The listing builds one solid part. Answer for the finished solid, in the listing's coordinates (mm). Face numbers are marked on the shaded views. A direction names the side the tool comes from. Give positions to 0.01 mm unless a question says otherwise; leave off trailing zeros. Loops run counter-clockwise (first coordinate to the right, second up) from the corner with the lowest first, then second, coordinate; pieces in that order, holes last.
Item 1: Section A-A, the plane x = 3 is taken. Give the vertices of the cut face in (y, z).
Item 2: Each of these flat-tipped pins is pushed along its axis until it touches: pin 1 Ø1 at (y, z) = (-10.5, -11.5) entering from -X; pin 2 Ø2 at (x, y) = (-3, 6.5) entering from +Z; pin 3 Ø3 at (x, z) = (-3.5, -9.5) entering from -Y; pin 4 Ø5 at (x, y) = (0, -9) entering from -Z. Where does it stop, or does it pass through?
Item 3: A tool of negligible diameter and unlimited length cuts with its end or side. For the marked faces 1 and 2, from which of +Z, -Z, +X, -X, +Y, -Y can it reach the whole face along a straight path? Write none if from no direction.
Item 4: The mould has two halves that part along Y. Classify the marked faces 3 and 4: pulls with the +Y half, pulls with the -Y half, needs draft (parallel to the pull), parting line crosses it, or undercut.
Item 5: Consider line 1 along Z through (x, y) = (1, 0); line 2 along X through (y, z) = (-9, 8.5); line 3 along Y through (x, z) = (2, 3). Determine where each line is inside the solid, lowest interval first.
Item 6: Section B-B, the plane z = 4 is taken. Give the number of separate pieces and of enclosed holes in the cut face, and give its area (3 significant figures).
Autodesk Inventor part; units mm, degrees
ref_plane "body_screw_XY" through (0, -9, 5) normal (0, 0, 1) x (1, 0, 0)
ref_plane "body_screw_YZ" through (0, -9, 5) normal (1, 0, 0) x (0, 1, 0)
ref_plane "body_screw_ZX" through (0, -9, 5) normal (0, 1, 0) x (0, 0, 1)
sketch "Sketch_1" plane through (0, 0, 0) normal (0, 0, 1) x (1, 0, 0)
  line L0 (5, 0) -> (-5, 0)
  line L1 (-5, 14.5) -> (-5, 5.5)
  line L2 (-5, 5.5) -> (-4.5, 5)
  line L3 (-4.5, 5) -> (4.5, 5)
  line L4 (4.5, 5) -> (5, 5.5)
  line L5 (5, 5.5) -> (5, 14.5)
  line L6 (5, 14.5) -> (4.5, 15)
  line L7 (4.5, 15) -> (-4.5, 15)
  line L8 (-4.5, 15) -> (-5, 14.5)
revolve "Revolution1" add sketch "Sketch_1" angle 360 about axis through (5, 0, 0) along (1, 0, 0)
sketch "Sketch_2" plane through (0, 0, 0) normal (1, 0, 0) x (0, 1, 0)
  line L0 (-15, 0.75) -> (-15, -0.75)
  line L1 (-15, -0.75) -> (9, -0.75)
  line L2 (9, -0.75) -> (9, 0.75)
  line L3 (9, 0.75) -> (-15, 0.75)
extrude "Extrusion1" cut sketch "Sketch_2" along normal mid plane 10
sketch "Sketch_3" plane through (0, 0, 0) normal (1, 0, 0) x (0, 1, 0)
  line L0 (-9, 15) -> (-9, 0)
  line L1 (-9, 0) -> (-11.25, 0)
  line L2 (-11.25, 0) -> (-11.25, 5)
  line L3 (-11.25, 5) -> (-12.75, 5)
  line L4 (-12.75, 5) -> (-12.75, 15)
  line L5 (-12.75, 15) -> (-9, 15)
  line L6 (-9, 15) -> (-9, 0)
revolve "Revolution2" cut sketch "Sketch_3" angle 360 about axis through (0, -9, 15) along (0, 0, 1)
sketch "Sketch_4" plane through (0, 0, 0) normal (1, 0, 0) x (0, 1, 0)
  line L0 (-9, -14.25) -> (-9, -0.75)
  line L1 (-9, -0.75) -> (-7, -0.75)
  line L2 (-7, -0.75) -> (-7.379, -1.129)
  line L3 (-7.379, -1.129) -> (-7.379, -14.25)
  line L4 (-7.379, -14.25) -> (-9, -14.25)
  line L5 (-9, -14.25) -> (-9, -0.75)
revolve "Revolution3" cut sketch "Sketch_4" angle 360 about axis through (0, -9, -14.25) along (0, 0, -1)
thread "Thread1"
sketch "Sketch_7" plane through (0, 0, -10) normal (0, 0, 1) x (1, 0, 0)
  line L0 (5, 0) -> (-5, 0)
  line L1 (-5, 0) -> (-5, 2.5)
  line L2 (-5, 2.5) -> (-4.567, 2.067)
  line L3 (-4.567, 2.067) -> (4.567, 2.067)
  line L4 (4.567, 2.067) -> (5, 2.5)
  line L5 (5, 2.5) -> (5, 0)
  line L6 (5, 0) -> (-5, 0)
revolve "Revolution4" cut sketch "Sketch_7" angle 360 about axis through (5, 0, -10) along (1, 0, 0)
thread "Thread2"
sketch "Sketch_8" plane through (0, 0, 10) normal (0, 0, 1) x (1, 0, 0)
  line L0 (5, 0) -> (-5, 0)
  line L1 (-5, 0) -> (-5, 2.5)
  line L2 (-5, 2.5) -> (-4.567, 2.067)
  line L3 (-4.567, 2.067) -> (4.567, 2.067)
  line L4 (4.567, 2.067) -> (5, 2.5)
  line L5 (5, 2.5) -> (5, 0)
  line L6 (5, 0) -> (-5, 0)
revolve "Revolution5" cut sketch "Sketch_8" angle 360 about axis through (5, 0, 10) along (1, 0, 0)
thread "Thread3"
ref_plane "body_screw_XY" through (0, -9, 5) normal (0, 0, 1) x (1, 0, 0)
ref_plane "body_screw_YZ" through (0, -9, 5) normal (1, 0, 0) x (0, 1, 0)
ref_plane "body_screw_ZX" through (0, -9, 5) normal (0, 1, 0) x (0, 0, 1)
properties part number "SSCSW10-10b"
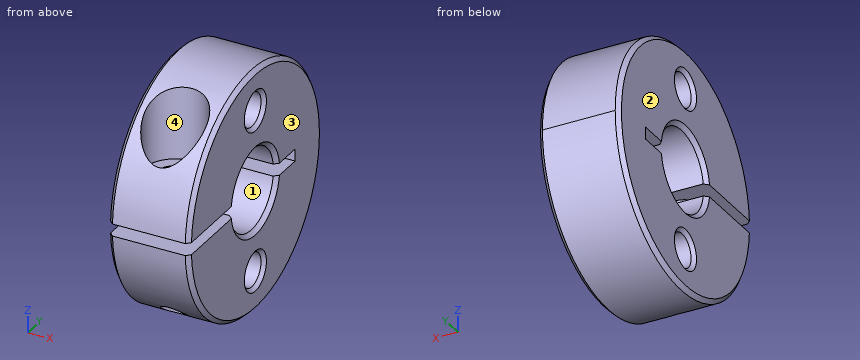
Worked answers:
1. outline: (-14.98, -0.75) arc R15 ccw (long way) to (-6.75, 13.4) - (-6.75, 5) - (-11.25, 5) - (-11.25, 9.92) arc R15 ccw to (-14.98, 0.75) - (-4.94, 0.75) arc R5 cw to (4.94, 0.75) - (9, 0.75) - (9, -0.75) - (4.94, -0.75) arc R5 cw to (-4.94, -0.75) - close; hole circle Ø4.13 at (0, -10); hole circle Ø4.13 at (0, 10)
2. pin 1: passes through
2. pin 2: stops at z = 13.96
2. pin 3: stops at y = -12.69
2. pin 4: stops at z = -13.52
3. face 1: +X, -X
3. face 2: +Z, -Z, -X, +Y, -Y
4. face 3: needs draft
4. face 4: undercut
5. line 1: z = -15 to -12.07, -7.93 to -5, 5 to 7.93, 12.07 to 15
5. line 2: x = -5 to -3.75, 3.75 to 5
5. line 3: y = -14.7 to -10.03, -7.97 to -4, 4 to 14.7
6. separate pieces: 2
6. enclosed holes: 1
6. area: 212 mm2
